Geometry check sheet. Reference: the model listing, model coordinates, mm. Round coordinates to 2 decimals unless told otherwise and drop trailing zeros. Loops run counter-clockwise (first coordinate to the right, second up) from the corner with the lowest first, then second, coordinate; pieces in that order, holes last. Notation, with made-up numbers: M -24,-9 L 24,-9 A31 cw 24,26 Z; hole C 73,58 d11. An arc over 180 degrees is marked long. Write item = value, one per line.
from build123d import *

# Parameters (mm, degrees)
SKETCH019_R          = 11
PAD015_DEPTH         = 5
SKETCH020_R          = 2.5
POCKET012_DEPTH      = 53.001
POCKET012_DEPTH_BACK = 1.797696
SKETCH021_R          = 2.5
POCKET013_DEPTH      = 1.297696
POCKET013_DEPTH_BACK = 53.501


with BuildPart() as part:
    # Sketch019 → Pad015 (new body, symmetric)
    with BuildSketch(Plane.XY):
        with BuildLine():
            ThreePointArc((-30.639841, 36.296696), (-33.587572, 33.587572), (-36.296696, 30.639841))
            Line((-36.296696, 30.639841), (-15.600467, 9.943613))
            ThreePointArc((-15.600467, 9.943613), (13.081475, -13.081475), (-9.943613, 15.600467))
            Line((-30.639841, 36.296696), (-9.943613, 15.600467))
        make_face()
        Circle(SKETCH019_R, mode=Mode.SUBTRACT)
    extrude(amount=PAD015_DEPTH, both=True)

    # Sketch020 → Pocket012 (cut, two sides)
    with BuildSketch(Plane(origin=(0, 34.5, 0), x_dir=(-1, 0, 0), z_dir=(0, 1, 0))) as pocket012_sk:
        Circle(SKETCH020_R)
    extrude(amount=-POCKET012_DEPTH, mode=Mode.SUBTRACT)
    extrude(pocket012_sk.sketch, amount=POCKET012_DEPTH_BACK, mode=Mode.SUBTRACT)

    # Sketch021 → Pocket013 (cut, two sides)
    with BuildSketch(Plane(origin=(-35, 0, 0), x_dir=(0, 0, -1), z_dir=(1, 0, 0))) as pocket013_sk:
        Circle(SKETCH021_R)
    extrude(amount=-POCKET013_DEPTH, mode=Mode.SUBTRACT)
    extrude(pocket013_sk.sketch, amount=POCKET013_DEPTH_BACK, mode=Mode.SUBTRACT)


solid = part.part
(1) Sectioned sample at A-A on x = 0. Record the cut outline in (y, z), then the cut area to 3 significant figures.
Result set:
outline = M -18.5,-5 L -11,-5 L -11,-2.5 L -18.5,-2.5 Z; M -18.5,2.5 L -11,2.5 L -11,5 L -18.5,5 Z; M 11,-5 L 18.5,-5 L 18.5,-2.5 L 11,-2.5 Z; M 11,2.5 L 18.5,2.5 L 18.5,5 L 11,5 Z
area = 75.0 mm2
(2) Release check for a two-part mould opening along X. For faces 1 (the cylindrical face through (14.55, -2.44, 0.54)), 2 (the cylindrical face through (0.54, -14.55, -2.44)), 3 (the cylindrical face through (-33.548, 33.627, 0.07)) record: released by +X, released by -X, zero draft, split by the parting line, or undercut.
Result set:
face_1 = zero draft
face_2 = undercut
face_3 = released by -X
(3) Material ranges on line 1 along Z through (x, y) = (0, 15.75); line 2 along Y through (x, z) = (-9, 3.75); line 3 along Y through (x, z) = (4, 2), recorded low to high. Write a range as from..to.
Result set:
line_1 = -5..-2.5, 2.5..5
line_2 = -16.16..-6.32, 6.32..16.16
line_3 = -18.06..-10.25, 10.25..18.06
(4) Sectioned sample at C-C on z = 3.75. Record the cut outline in (x, y).
Result set:
outline = M -36.3,30.64 L -15.6,9.94 A18.5 ccw long -9.94,15.6 L -30.64,36.3 A47.5 ccw Z; hole C 0,0 d22
(5) Depth check by flat-ended pin: pin 1 Ø3 at (x, z) = (0, 0) entering from -Y; pin 2 Ø6 at (x, y) = (-3, 9) entering from -Z; pin 3 Ø2 at (x, z) = (-26, -3) entering from -Y; pin 4 Ø4 at (y, z) = (27, 1.5) entering from -X. Enter the tip coordinate at first touch or a pass-through.
Result set:
pin_1 = through
pin_2 = -5
pin_3 = 19.34
pin_4 = -34.66
(6) Sectioned sample at D-D on z = 0. Record the cut outline in (x, y), then the cut area to 3 significant figures.
Result set:
outline = M -36.3,30.64 L -15.6,9.94 A18.5 ccw -18.33,2.5 L -10.71,2.5 A11 cw -2.5,10.71 L -2.5,18.33 A18.5 ccw -9.94,15.6 L -30.64,36.3 A47.5 ccw Z; M -18.33,-2.5 A18.5 ccw -2.5,-18.33 L -2.5,-10.71 A11 cw -10.71,-2.5 Z; M 2.5,-18.33 A18.5 ccw 18.33,-2.5 L 10.71,-2.5 A11 cw 2.5,-10.71 Z; M 2.5,10.71 A11 cw 10.71,2.5 L 18.33,2.5 A18.5 ccw 2.5,18.33 Z
area = 777 mm2
